```python
from build123d import *

# Parameters (mm, degrees)
F0_W     = 255
F0_H     = 405
F0_W_2   = 120
F0_H_2   = 30
F1_DEPTH = 10
F2_R     = 10


with BuildPart() as f1:
    # F0 (on Top) → F1 (new body)
    with BuildSketch(Plane.XY):
        Rectangle(F0_W, F0_H)
        with Locations((0, 157.5)):
            Rectangle(F0_W_2, F0_H_2, mode=Mode.SUBTRACT)
    extrude(amount=F1_DEPTH)

    # F2
    f2_edges = [f1.edges().sort_by_distance(p)[0] for p in [
        (-127.5, 202.5, 5),
        (127.5, 202.5, 5),
        (60, 142.5, 5),
        (60, 172.5, 5),
        (-60, 172.5, 5),
        (-60, 142.5, 5),
        (127.5, -202.5, 5),
        (-127.5, -202.5, 5),
    ]]
    fillet(f2_edges, radius=F2_R)


solid = f1.part
```
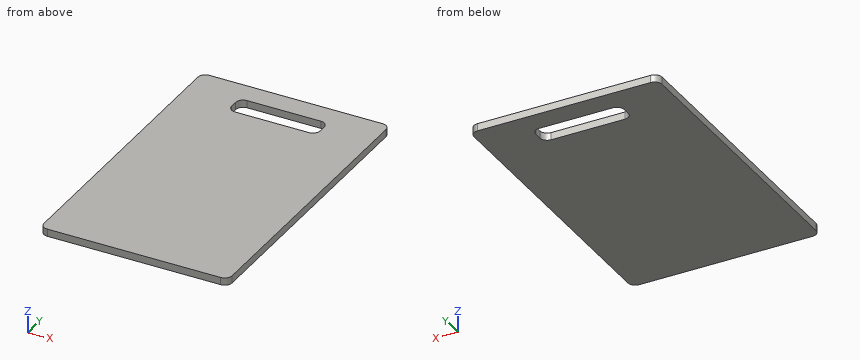
Work out the finished part from the listing and answer in its coordinate system (mm). Give positions to 0.01 mm unless a question says otherwise; leave off trailing zeros. Order: outer loops, then holes, each group sorted by start corner. A loop starts at its lowest first (then second) coordinate and runs counter-clockwise, first axis right, second up. Notation, with made-up numbers: (26.25, 73) - (51.25, 73) arc R21 cw to (51.25, 79) - close; hole circle Ø7 at (14, 71.25). An arc over 180 degrees is marked (long way). One line per item, written item: value. Start each with the question number.
1. Section B-B, the plane z = 2 is taken. Write down the section's boundary in (x, y).
2. Section A-A, the plane x = -32.5 is taken. Write down the section's boundary in (y, z), then the cut area to 3 significant figures.
3. Consider line 1 (Y direction, x = 25, z = 2.25); line 2 (X direction, y = 150, z = 7.5). Determine where each line is inside the solid, lowest interval first.
Filled sheet:
1. outline: (-127.5, -192.5) arc R10 ccw to (-117.5, -202.5) - (117.5, -202.5) arc R10 ccw to (127.5, -192.5) - (127.5, 192.5) arc R10 ccw to (117.5, 202.5) - (-117.5, 202.5) arc R10 ccw to (-127.5, 192.5) - close; hole (-60, 152.5) arc R10 ccw to (-50, 142.5) - (50, 142.5) arc R10 ccw to (60, 152.5) - (60, 162.5) arc R10 ccw to (50, 172.5) - (-50, 172.5) arc R10 ccw to (-60, 162.5) - close
2. outline: (-202.5, 0) - (142.5, 0) - (142.5, 10) - (-202.5, 10) - close; (172.5, 0) - (202.5, 0) - (202.5, 10) - (172.5, 10) - close
2. area: 3,750 mm²
3. line 1: -202.5 to 142.5, 172.5 to 202.5
3. line 2: -127.5 to -59.68, 59.68 to 127.5
